from build123d import *

# Parameters (mm, degrees)
SKETCH_R  = 2
PAD_DEPTH = 5


with BuildPart() as part:
    # Sketch → Pad (new body)
    with BuildSketch(Plane.XY):
        with BuildLine():
            ThreePointArc((7.893378, 21.767666), (10, 17.25), (12.106622, 21.767666))
            ThreePointArc((14.404756, 23.696029), (12.291507, 23.880914), (12.106622, 21.767666))
            ThreePointArc((15, 22.839454), (14.721841, 23.281267), (14.404756, 23.696029))
            ThreePointArc((15.595244, 23.696029), (15.278159, 23.281267), (15, 22.839454))
            ThreePointArc((17.893378, 21.767666), (17.708493, 23.880914), (15.595244, 23.696029))
            ThreePointArc((17.893378, 21.767666), (20, 17.25), (22.106622, 21.767666))
            ThreePointArc((24.404756, 23.696029), (22.291507, 23.880914), (22.106622, 21.767666))
            ThreePointArc((25, 22.839454), (24.721841, 23.281267), (24.404756, 23.696029))
            ThreePointArc((25.595244, 23.696029), (25.278159, 23.281267), (25, 22.839454))
            ThreePointArc((27.893378, 21.767666), (27.708493, 23.880914), (25.595244, 23.696029))
            ThreePointArc((27.893378, 21.767666), (30, 17.25), (32.106622, 21.767666))
            ThreePointArc((34.404756, 23.696029), (32.291507, 23.880914), (32.106622, 21.767666))
            ThreePointArc((35, 22.839454), (34.721841, 23.281267), (34.404756, 23.696029))
            ThreePointArc((35.595244, 23.696029), (35.278159, 23.281267), (35, 22.839454))
            ThreePointArc((37.893378, 21.767666), (37.708493, 23.880914), (35.595244, 23.696029))
            ThreePointArc((37.893378, 21.767666), (40, 17.25), (42.106622, 21.767666))
            ThreePointArc((44.404756, 23.696029), (42.291507, 23.880914), (42.106622, 21.767666))
            ThreePointArc((42.839454, 15), (45.659052, 18.98136), (44.404756, 23.696029))
            ThreePointArc((44.404756, 6.303971), (45.659052, 11.01864), (42.839454, 15))
            ThreePointArc((42.106622, 8.232334), (42.291507, 6.119086), (44.404756, 6.303971))
            ThreePointArc((42.106622, 8.232334), (40, 12.75), (37.893378, 8.232334))
            ThreePointArc((35.595244, 6.303971), (37.708493, 6.119086), (37.893378, 8.232334))
            ThreePointArc((35, 7.160546), (35.278159, 6.718733), (35.595244, 6.303971))
            ThreePointArc((34.404756, 6.303971), (34.721841, 6.718733), (35, 7.160546))
            ThreePointArc((32.106622, 8.232334), (32.291507, 6.119086), (34.404756, 6.303971))
            ThreePointArc((32.106622, 8.232334), (30, 12.75), (27.893378, 8.232334))
            ThreePointArc((25.595244, 6.303971), (27.708493, 6.119086), (27.893378, 8.232334))
            ThreePointArc((25, 7.160546), (25.278159, 6.718733), (25.595244, 6.303971))
            ThreePointArc((24.404756, 6.303971), (24.721841, 6.718733), (25, 7.160546))
            ThreePointArc((22.106622, 8.232334), (22.291507, 6.119086), (24.404756, 6.303971))
            ThreePointArc((22.106622, 8.232334), (20, 12.75), (17.893378, 8.232334))
            ThreePointArc((15.595244, 6.303971), (17.708493, 6.119086), (17.893378, 8.232334))
            ThreePointArc((15, 7.160546), (15.278159, 6.718733), (15.595244, 6.303971))
            ThreePointArc((14.404756, 6.303971), (14.721841, 6.718733), (15, 7.160546))
            ThreePointArc((12.106622, 8.232334), (12.291507, 6.119086), (14.404756, 6.303971))
            ThreePointArc((12.106622, 8.232334), (10, 12.75), (7.893378, 8.232334))
            ThreePointArc((5.595244, 6.303971), (7.708493, 6.119086), (7.893378, 8.232334))
            ThreePointArc((7.160546, 15), (4.340948, 11.01864), (5.595244, 6.303971))
            ThreePointArc((5.595244, 23.696029), (4.340948, 18.98136), (7.160546, 15))
            ThreePointArc((7.893378, 21.767666), (7.708493, 23.880914), (5.595244, 23.696029))
        make_face()
        with Locations((15, 15)):
            Circle(SKETCH_R, mode=Mode.SUBTRACT)
        with Locations((25, 15)):
            Circle(SKETCH_R, mode=Mode.SUBTRACT)
        with Locations((35, 15)):
            Circle(SKETCH_R, mode=Mode.SUBTRACT)
    extrude(amount=PAD_DEPTH)


solid = part.part
Geometry check sheet. Reference: the model listing, model coordinates, mm. Give positions to 0.01 mm unless a question says otherwise; leave off trailing zeros. Order: outer loops, then holes, each group sorted by start corner. A loop starts at its lowest first (then second) coordinate and runs counter-clockwise, first axis right, second up.
1. Sectioned sample at A-A (y = 10). Record the boundary of the cut face in (x, z).
Completed:
outline: (4.25, 0) - (7.25, 0) - (7.25, 5) - (4.25, 5) - close; (12.75, 0) - (17.25, 0) - (17.25, 5) - (12.75, 5) - close; (22.75, 0) - (27.25, 0) - (27.25, 5) - (22.75, 5) - close; (32.75, 0) - (37.25, 0) - (37.25, 5) - (32.75, 5) - close; (42.75, 0) - (45.75, 0) - (45.75, 5) - (42.75, 5) - close
2. Sectioned sample at B-B (x = 34). Record the boundary of the cut face in (y, z), then the cut area to 3 significant figures.
Completed:
outline: (5.97, 0) - (13.27, 0) - (13.27, 5) - (5.97, 5) - close; (16.73, 0) - (24.03, 0) - (24.03, 5) - (16.73, 5) - close
area: 73.0 mm2
3. Depth check by flat-ended pin: pin 1 (5 mm diameter, centred on x = 40, y = 20, fed in from +Z); pin 2 (1.5 mm diameter, centred on x = 28.5, z = 4, fed in from +Y); pin 3 (1 mm diameter, centred on x = 15.5, z = 3.5, fed in from +Y). Enter the tip coordinate at first touch or a pass-through.
Completed:
pin 1: passes through
pin 2: stops at y = 23.84
pin 3: stops at y = 24.03
4. Scan lines: line 1 (X direction, y = 10, z = 1.6); line 2 (X direction, y = 16.5, z = 3.65); line 3 (X direction, y = 8.25, z = 3.15). Record each from-to range of solid material in increasing order.
Completed:
line 1: x = 4.25 to 7.25, 12.75 to 17.25, 22.75 to 27.25, 32.75 to 37.25, 42.75 to 45.75
line 2: x = 5.44 to 13.68, 16.32 to 23.68, 26.32 to 33.68, 36.32 to 44.56
line 3: x = 4.52 to 7.88, 12.12 to 17.88, 22.12 to 27.88, 32.12 to 37.88, 42.12 to 45.48
5. Draft check along Y on faces 1 (the face through (25.3, 17.2, 0)), 2 (the face through (30.09, 12.75, 2.46)). Enter one of: pulls with the +Y half, pulls with the -Y half, needs draft (parallel to the pull), parting line crosses it, or undercut.
Completed:
face 1: needs draft
face 2: undercut
6. Sectioned sample at D-D (x = 40). Record the boundary of the cut face in (y, z), then the cut area to 3 significant figures.
Completed:
outline: (12.75, 0) - (17.25, 0) - (17.25, 5) - (12.75, 5) - close
area: 22.5 mm2
7. Sectioned sample at C-C (y = 12.25). Record the boundary of the cut face in (x, z), then the cut area to 3 significant figures.
Completed:
outline: (4.71, 0) - (8.42, 0) - (8.42, 5) - (4.71, 5) - close; (11.58, 0) - (18.42, 0) - (18.42, 5) - (11.58, 5) - close; (21.58, 0) - (28.42, 0) - (28.42, 5) - (21.58, 5) - close; (31.58, 0) - (38.42, 0) - (38.42, 5) - (31.58, 5) - close; (41.58, 0) - (45.29, 0) - (45.29, 5) - (41.58, 5) - close
area: 140 mm2
